from build123d import *

# Parameters (mm, degrees)
SKETCH1_W           = 10
SKETCH1_H           = 10
BOSS_EXTRUDE1_DEPTH = 2.5
BOSS_EXTRUDE2_DEPTH = 3.5


with BuildPart() as part:
    # Sketch1 → Boss-Extrude1 (new body)
    with BuildSketch(Plane(origin=(0, 0, 0), x_dir=(1, 0, 0), z_dir=(0, 1, 0))):
        Rectangle(SKETCH1_W, SKETCH1_H)
        with BuildLine():
            ThreePointArc((-1.44, 1.625), (-3.065, 0), (-1.44, -1.625))
            Line((-1.44, -1.625), (1.44, -1.625))
            ThreePointArc((1.44, -1.625), (3.065, 0), (1.44, 1.625))
            Line((1.44, 1.625), (-1.44, 1.625))
        make_face(mode=Mode.SUBTRACT)
    extrude(amount=BOSS_EXTRUDE1_DEPTH)

    # Sketch2 → Boss-Extrude2 (add)
    with BuildSketch(Plane(origin=(0, 2.5, 0), x_dir=(1, 0, 0), z_dir=(0, 1, 0))):
        Polygon((-5, -5), (-5, 5), (5, 5), (5, -5), (6, -5), (6, 6), (-6, 6), (-6, -5), align=None)
    extrude(amount=-BOSS_EXTRUDE2_DEPTH)


solid = part.part
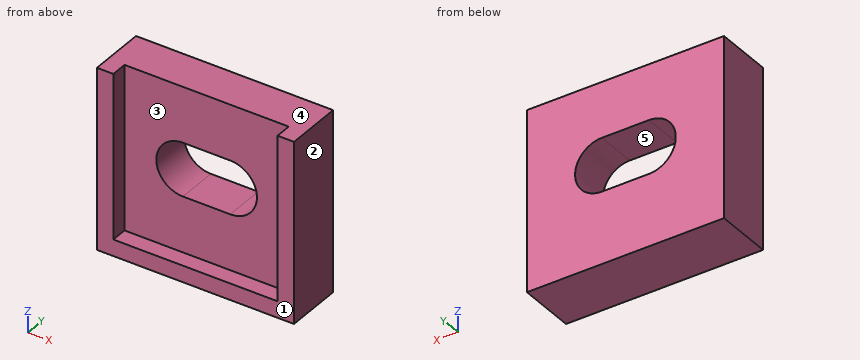
Work out the finished part from the listing and answer in its coordinate system (mm). Face numbers are marked on the shaded views. A direction names the side the tool comes from. Give positions to 0.01 mm unless a question says otherwise; leave off trailing zeros. Loops run counter-clockwise (first coordinate to the right, second up) from the corner with the lowest first, then second, coordinate; pieces in that order, holes last. Notation, with made-up numbers: (78, -19) -> (118, -19) arc R28 ccw to (118, 17) -> close; hole circle Ø2 at (-15, 88). An arc over 180 degrees is marked (long way). Use a Markdown table: item, result. Add a question column.
1) For a pull along X with two mould halves and no side action, classify the marked faces 1, 2 and 3 as +X half, -X half, draft (parallel to the pull), parting line (faces both ways), or undercut.
2) Which of the six approach directions +Z, -Z, +X, -X, +Y, -Y give full straight-line access (tool end or side, diameter ignored) to the marked faces 4 and 5?
3) The part is cut by section C-C, the plane y = -0.15. Determine the outline of the cut face in (x, z), plus the area to 3 significant figures.
4) Consider line 1 along X through (y, z) = (-0.7, -2.75); line 2 along Z through (x, y) = (-1.5, 0.85); line 3 along Z through (x, y) = (-1.75, -0.6). Determine where each line is inside the solid, lowest interval first.
5) The part is cut by section B-B, the plane x = 1. Determine the outline of the cut face in (y, z) (3 decimals), plus the area to 3 significant figures.
6) The part is cut by section D-D, the plane y = 1.95. Determine the outline of the cut face in (x, z) (3 decimals), plus the area to 3 significant figures.
7) The part is cut by section A-A, the plane z = 0. Determine the outline of the cut face in (x, y) (3 decimals), plus the area to 3 significant figures.
8) Each of these flat-tipped pins is pushed along its axis until it touches: P1, Ø0.5, axis at x = 0, y = -0.5, coming from the +Z side; P2, Ø5, axis at x = -1.5, z = 1, coming from the -Y side. Where does it stop, or does it pass through?
Reported:
| question | item | result |
|---|---|---|
| 1 | face 1 | draft |
| 1 | face 2 | +X half |
| 1 | face 3 | undercut |
| 2 | face 4 | +Z, +X, -X, +Y, -Y |
| 2 | face 5 | +Y, -Y |
| 3 | outline | (-6, -6) -> (6, -6) -> (6, 5) -> (5, 5) -> (5, -5) -> (-5, -5) -> (-5, 5) -> (-6, 5) -> close |
| 3 | area | 32.0 mm^2 |
| 4 | line 1 | x = -6 to -5, 5 to 6 |
| 4 | line 2 | z = -6 to -1.62, 1.62 to 5 |
| 4 | line 3 | z = -6 to -5 |
| 5 | outline | (-1, -6) -> (2.5, -6) -> (2.5, -1.625) -> (0, -1.625) -> (0, -5) -> (-1, -5) -> close; (0, 1.625) -> (2.5, 1.625) -> (2.5, 5) -> (0, 5) -> close |
| 5 | area | 20.4 mm^2 |
| 6 | outline | (-6, -6) -> (6, -6) -> (6, 5) -> (-6, 5) -> close; hole (-1.44, -1.625) -> (1.44, -1.625) arc R1.625 ccw to (1.44, 1.625) -> (-1.44, 1.625) arc R1.625 ccw to start |
| 6 | area | 114 mm^2 |
| 7 | outline | (-6, -1) -> (-5, -1) -> (-5, 0) -> (-3.065, 0) -> (-3.065, 2.5) -> (-6, 2.5) -> close; (3.065, 0) -> (5, 0) -> (5, -1) -> (6, -1) -> (6, 2.5) -> (3.065, 2.5) -> close |
| 7 | area | 16.7 mm^2 |
| 8 | P1 | stops at z = -5 |
| 8 | P2 | stops at y = 0 |
